CAD build for the part. Positions are in the model's coordinates, mm. A direction names the side the tool comes from. Give positions to 0.01 mm unless a question says otherwise; leave off trailing zeros. Loops run counter-clockwise (first coordinate to the right, second up) from the corner with the lowest first, then second, coordinate; pieces in that order, holes last.
Item 1: Saw through at B-B on y = 7. Give the cut face in (x, z).
Item 2: Saw through at C-C on x = -4. Give the cut face in (y, z), plus the area to 3 significant figures.
Item 3: Probe probe 1 along X at (y, z) = (4.5, 0); probe 2 along Z at (x, y) = (0, 1.5); probe 3 along X at (y, z) = (4.5, 2). List the from-to ranges inside material, lowest first.
Item 4: Which spindle directions (+Z, -Z, +X, -X, +Y, -Y) get a long thin tool onto all of the face, cutting with end or side? Do faces 5 (the flat face through (7, 4, 14.5)), 6 (the cylindrical face through (27, 4, 0)). Say none if no direction does.
Item 5: Saw through at D-D on z = -8.5. Give the cut face in (x, y).
Item 6: Mould opens along Z. For faces 1 (the flat face through (7, 4, -14.5)), 2 (the cylindrical face through (29, 4, 0)), 3 (the cylindrical face through (11.923, 3.944, -3.755)), 4 (the flat face through (14.5, 4, 0)) say: released by +Z, released by -Z, zero draft, split by the parting line, or undercut.
Item 7: Drop flat-ended pins along their axis: P1, Ø4, axis at y = 4.5, z = -5, coming from the +X side; P2, Ø3, axis at y = 5, z = -2.5, coming from the -X side; P3, Ø4, axis at y = 4, z = 4.5, coming from the -X side. Give the stop position or say it passes through.
Item 8: Saw through at A-A on z = 0. Give the cut face in (x, y).
from build123d import *

# Parameters (mm, degrees)
SKETCH_1_R      = 12.5
EXTRUDE_1_DEPTH = 8
EXTRUDE_2_DEPTH = 8


with BuildPart() as part:
    # Sketch 1 → Extrude 1 (new body)
    with BuildSketch(Plane(origin=(0, 0, 0), x_dir=(1, 0, 0), z_dir=(0, 1, 0))):
        with BuildLine():
            Line((0, -14.5), (14.5, -14.5))
            Line((14.5, -14.5), (14.5, 14.5))
            Line((14.5, 14.5), (0, 14.5))
            ThreePointArc((0, 14.5), (-14.5, 0), (0, -14.5))
        make_face()
        Circle(SKETCH_1_R, mode=Mode.SUBTRACT)
    extrude(amount=EXTRUDE_1_DEPTH)

    # Sketch 1_3 → Extrude 2 (add)
    with BuildSketch(Plane(origin=(0, 0, 0), x_dir=(1, 0, 0), z_dir=(0, 1, 0))):
        with BuildLine():
            Line((14.5, -12.5), (14.5, -14.5))
            ThreePointArc((14.5, -14.5), (29, 0), (14.5, 14.5))
            Line((14.5, 14.5), (14.5, 12.5))
            ThreePointArc((14.5, 12.5), (27, 0), (14.5, -12.5))
        make_face()
    extrude(amount=EXTRUDE_2_DEPTH)


solid = part.part
Results below:
1. outline: (0, -14.5) - (14.5, -14.5) arc R14.5 ccw to (14.5, 14.5) - (0, 14.5) arc R14.5 ccw to start; hole circle Ø25 at (0, 0); hole (14.5, -12.5) arc R12.5 ccw to (14.5, 12.5) - close
2. outline: (0, -13.94) - (8, -13.94) - (8, -11.84) - (0, -11.84) - close; (0, 11.84) - (8, 11.84) - (8, 13.94) - (0, 13.94) - close
2. area: 33.5 mm2
3. probe 1: x = -14.5 to -12.5, 12.5 to 14.5, 27 to 29
3. probe 2: z = -14.5 to -12.5, 12.5 to 14.5
3. probe 3: x = -14.36 to -12.34, 12.34 to 14.5, 26.84 to 28.86
4. face 5: +Z, +X, -X, +Y, -Y
4. face 6: +Y, -Y
5. outline: (-11.75, 0) - (-9.17, 0) - (-9.17, 8) - (-11.75, 8) - close; (9.17, 0) - (14.5, 0) - (14.5, 8) - (9.17, 8) - close; (23.67, 0) - (26.25, 0) - (26.25, 8) - (23.67, 8) - close
6. face 1: released by -Z
6. face 2: split by the parting line
6. face 3: undercut
6. face 4: undercut
7. P1: stops at x = 28.69
7. P2: stops at x = -14.47
7. P3: stops at x = -14.28
8. outline: (-14.5, 0) - (-12.5, 0) - (-12.5, 8) - (-14.5, 8) - close; (12.5, 0) - (14.5, 0) - (14.5, 8) - (12.5, 8) - close; (27, 0) - (29, 0) - (29, 8) - (27, 8) - close
